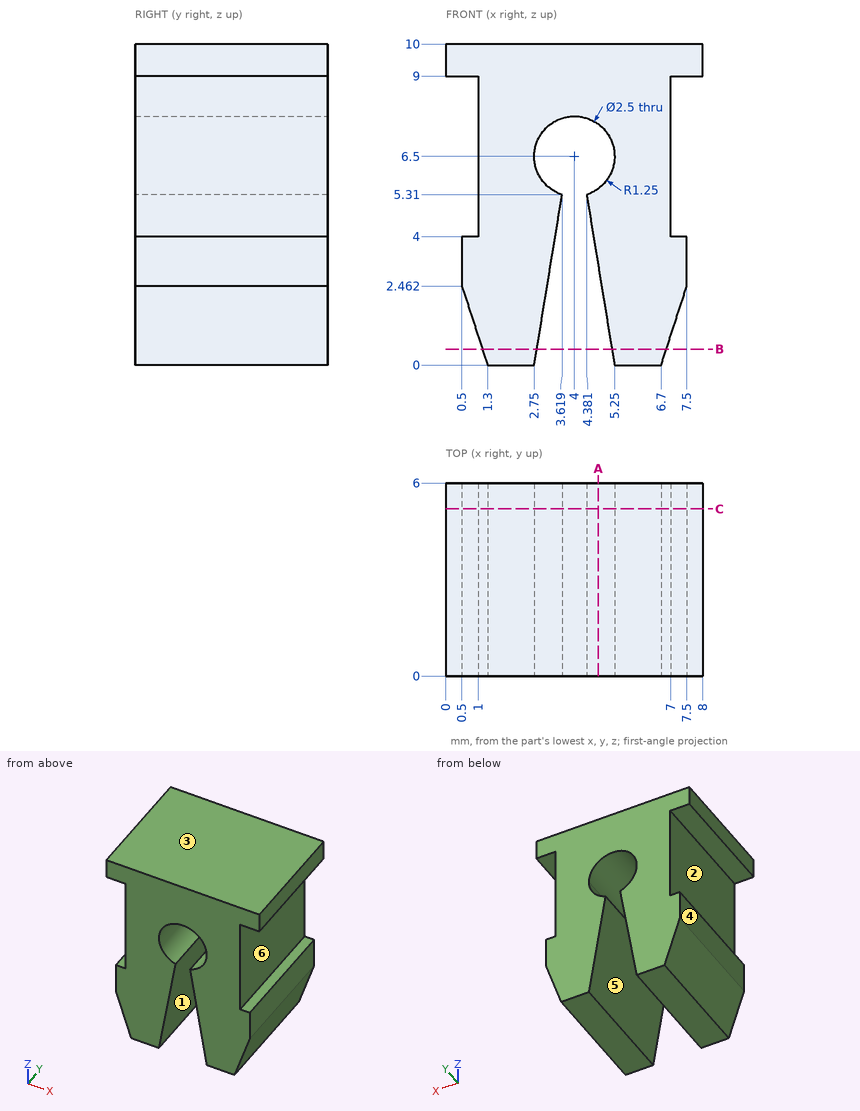
For this review, use the dimensioned drawing (mm, ordinates from the lowest corner) and the shaded views. A direction names the side the tool comes from. Coordinates: 2 decimals unless noted, no trailing zeros. Loops run counter-clockwise (first coordinate to the right, second up) from the corner with the lowest first, then second, coordinate; pieces in that order, holes last. Notation, with made-up numbers: (81.25, 40) - (140.25, 40) arc R18 cw to (140.25, 68) - close; hole circle Ø1 at (-32.5, -7). An arc over 180 degrees is marked (long way). Use CSV: the item, a comma, the result in double quotes. Start each with the question number.
1) Wall thickness on L1, parallel to Z at x = 4, y = 1.4; L2, parallel to X at y = 3.65, z = 2.25; L3, parallel to X at y = 2.85, z = 8.5: over which ranges is each line inside the solid? List them lowest first. Write a range as from..to.
2) Consider section B-B on z = 0.5. Write out the cut boundary in (x, y).
3) Tool access review of the marked faces 4, 5 and 6: name each direction out of +Z, -Z, +X, -X, +Y, -Y from which nothing blocks a thin tool from reaching the whole face with its end or side.
4) For pin 1 Ø2 at (x, y) = (3.5, 5.5) entering from -Z; pin 2 Ø1.5 at (y, z) = (1, 1) entering from +X; pin 3 Ø0.8 at (y, z) = (4.5, 3.5) entering from -X; pin 4 Ø0.5 at (y, z) = (4, 3.5) entering from +X, all flat-tipped, find the tip position at first contact; note any pin that passes through.
5) Consider section A-A on x = 4.75. Write out the cut boundary in (y, z) (1 decimal).
6) The part is to be moulded in two halves that separate along X. For the marked faces 1, 2 and 3, say which applies: +X half, -X half, draft (parallel to the pull), parting line (faces both ways), or undercut.
7) Consider section C-C on y = 5.2. Write out the cut boundary in (x, z).
Geometry says:
1,L1,"7.75..10"
1,L2,"0.57..3.12, 4.88..7.43"
1,L3,"1..7"
2,outline,"(1.14, 0) - (2.83, 0) - (2.83, 6) - (1.14, 6) - close; (5.17, 0) - (6.86, 0) - (6.86, 6) - (5.17, 6) - close"
3,face 4,"-Z, -X, +Y, -Y"
3,face 5,"-Z, +Y, -Y"
3,face 6,"+X, +Y, -Y"
4,pin 1,"z = 0"
4,pin 2,"x = 7.27"
4,pin 3,"x = 0.5"
4,pin 4,"x = 7.5"
5,outline,"(0, 3.1) - (6, 3.1) - (6, 5.5) - (0, 5.5) - close; (0, 7.5) - (6, 7.5) - (6, 10) - (0, 10) - close"
6,face 1,"undercut"
6,face 2,"-X half"
6,face 3,"draft"
7,outline,"(0, 9) - (1, 9) - (1, 4) - (0.5, 4) - (0.5, 2.46) - (1.3, 0) - (2.75, 0) - (3.62, 5.31) arc R1.25 cw (long way) to (4.38, 5.31) - (5.25, 0) - (6.7, 0) - (7.5, 2.46) - (7.5, 4) - (7, 4) - (7, 9) - (8, 9) - (8, 10) - (0, 10) - close"
